For this review, take the finished solid that the model builds, in its own axes (mm). A direction names the side the tool comes from. Give positions to 0.01 mm unless a question says otherwise; leave off trailing zeros. Write each loop counter-clockwise with the first axis right and the second up, starting at its lowest first coordinate (ties: lowest second). Pieces come first, ordered by that corner, then holes. Notation, with made-up numbers: (49.25, 4.5) -> (76.25, 4.5) arc R20 cw to (76.25, 37.5) -> close; hole circle Ø7 at (63, 40). An arc over 180 degrees is marked (long way). Write item = value, one per line.
```python
from build123d import *

# Parameters (mm, degrees)
SKETCH1_W           = 4.5
SKETCH1_H           = 4.5
BOSS_EXTRUDE1_DEPTH = 6
SKETCH2_W           = 3.2
SKETCH2_H           = 3.2
CUT_EXTRUDE1_DEPTH  = 4.9
CUT_EXTRUDE2_DEPTH  = 4.5
LPATTERN1_COUNT     = 5
LPATTERN1_PITCH     = 0.725
CHAMFER1_SIZE       = 0.3


with BuildPart() as part:
    # Sketch1 → Boss-Extrude1 (new body)
    with BuildSketch(Plane(origin=(0, 0, 0), x_dir=(1, 0, 0), z_dir=(0, 1, 0))):
        with Locations((2.25, 2.25)):
            Rectangle(SKETCH1_W, SKETCH1_H)
    extrude(amount=BOSS_EXTRUDE1_DEPTH)

    # Sketch2 → Cut-Extrude1 (cut)
    with BuildSketch(Plane.XZ):
        with Locations((2.25, -2.25)):
            Rectangle(SKETCH2_W, SKETCH2_H)
    extrude(amount=-CUT_EXTRUDE1_DEPTH, mode=Mode.SUBTRACT)

    # Sketch3 → Cut-Extrude2 (cut)
    with BuildSketch(Plane.ZY):
        Polygon((-4, 6), (-3.7, 5.33), (-3.4, 6), align=None)
    cut_extrude2 = extrude(amount=-CUT_EXTRUDE2_DEPTH, mode=Mode.SUBTRACT)

    # LPattern1: Cut-Extrude2 ×5
    with Locations(*[(0, 0, i * LPATTERN1_PITCH) for i in range(1, LPATTERN1_COUNT)]):
        add(cut_extrude2, mode=Mode.SUBTRACT)

    # Chamfer1
    chamfer1_edges = [part.edges().sort_by_distance(p)[0] for p in [
        (4.5, 6, -0.25),
        (2.25, 6, -4.5),
        (4.5, 6, -4.25),
        (0, 6, -0.25),
        (0, 6, -4.25),
        (2.25, 6, 0),
    ]]
    chamfer(chamfer1_edges, length=CHAMFER1_SIZE)


solid = part.part
```
(1) Take a section at C-C (y = 5.45). Write out the cut boundary in (x, z).
Answers below:
outline = (0, -4.5) -> (4.5, -4.5) -> (4.5, -3.75) -> (0, -3.75) -> close; (0, -3.65) -> (4.5, -3.65) -> (4.5, -3.03) -> (0, -3.03) -> close; (0, -2.92) -> (4.5, -2.92) -> (4.5, -2.3) -> (0, -2.3) -> close; (0, -2.2) -> (4.5, -2.2) -> (4.5, -1.58) -> (0, -1.58) -> close; (0, -1.47) -> (4.5, -1.47) -> (4.5, -0.85) -> (0, -0.85) -> close; (0, -0.75) -> (4.5, -0.75) -> (4.5, 0) -> (0, 0) -> close
(2) Take a section at D-D (z = -2.4). Write out the cut boundary in (x, y) (3 decimals).
Answers below:
outline = (0, 0) -> (0.65, 0) -> (0.65, 4.9) -> (3.85, 4.9) -> (3.85, 0) -> (4.5, 0) -> (4.5, 5.665) -> (0, 5.665) -> close
(3) To check wall thickness, follow probe 1 along Z at (x, y) = (1.15, 3.2); probe 2 along Z at (x, y) = (4.15, 5.65); probe 3 along X at (y, z) = (4.15, -3.65). State the ranges of each line that lie inside material, in increasing order.
Answers below:
probe_1 = -4.5 to -3.85, -0.65 to 0
probe_2 = -4.5 to -3.84, -3.56 to -3.12, -2.83 to -2.39, -2.11 to -1.67, -1.38 to -0.94, -0.66 to 0
probe_3 = 0 to 0.65, 3.85 to 4.5
(4) For pin 1 (2.5 mm diameter, centred on x = 2, z = -3, fed in from -Y), flat-tipped, find the tip position at first contact; note if it passes through.
Answers below:
pin_1 = 0
(5) Tool access review of faces 1 (the face through (4.5, 3, -2)), 2 (the face through (2, 4.9, -2)): name each direction out of +Z, -Z, +X, -X, +Y, -Y from which nothing blocks a thin tool from reaching the whole face with its end or side.
Answers below:
face_1 = +Z, -Z, +X, +Y, -Y
face_2 = -Y
(6) Take a section at A-A (y = 3.1). Write out the cut boundary in (x, z), plus the area to 3 significant figures.
Answers below:
outline = (0, -4.5) -> (4.5, -4.5) -> (4.5, 0) -> (0, 0) -> close; hole (0.65, -3.85) -> (3.85, -3.85) -> (3.85, -0.65) -> (0.65, -0.65) -> close
area = 10.0 mm^2
(7) Take a section at B-B (x = 3.95). Write out the cut boundary in (y, z) (3 decimals), plus the area to 3 significant figures.
Answers below:
outline = (0, -4.5) -> (5.7, -4.5) -> (6, -4.2) -> (6, -4) -> (5.33, -3.7) -> (6, -3.4) -> (6, -3.275) -> (5.33, -2.975) -> (6, -2.675) -> (6, -2.55) -> (5.33, -2.25) -> (6, -1.95) -> (6, -1.825) -> (5.33, -1.525) -> (6, -1.225) -> (6, -1.1) -> (5.33, -0.8) -> (6, -0.5) -> (6, -0.3) -> (5.7, 0) -> (0, 0) -> close
area = 25.9 mm^2
(8) The part is to be moulded in two halves that separate along X. For faces 3 (the face through (2, 2, -0.65)), 4 (the face through (0, 3, -2)), 5 (the face through (3.85, 2, -2)), 6 (the face through (4.2, 0, -2.3)), say which applies: released by +X, released by -X, zero draft, split by the parting line, or undercut.
Answers below:
face_3 = undercut
face_4 = released by -X
face_5 = undercut
face_6 = zero draft
